Geometry check sheet. Reference: the model listing, model coordinates, mm. Face numbers are marked on the shaded views. A direction names the side the tool comes from. Give positions to 0.01 mm unless a question says otherwise; leave off trailing zeros. Write each loop counter-clockwise with the first axis right and the second up, starting at its lowest first coordinate (ties: lowest second). Pieces come first, ordered by that corner, then holes.
(1) Depth check by flat-ended pin: P1, Ø0.6, axis at y = 10.5, z = 3.5, coming from the -X side; P2, Ø5, axis at x = -6.5, y = 5, coming from the +Z side. Enter the tip coordinate at first touch or a pass-through.
(2) Tool access check on the marked faces 1, 2, 3, 4 and 5. Record the directions out of +Z, -Z, +X, -X, +Y, -Y that give a thin tool (end or side, any length) a straight path to the whole face; none if there is none.
(3) Cross-section at C-C (y = 10.5). Count the separate pieces of the cut face and the enclosed holes in it, and give its area (3 significant figures).
(4) Thickness scan on line 1 along Y through (x, z) = (7.62, 3.35) (3 decimals); line 2 along X through (y, z) = (-4, 2.65); line 3 along X through (y, z) = (8.75, 0.3). Record the ranges inside material, lowest first.
(5) Cross-section at A-A (x = 0). Record the boundary of the cut face in (y, z) (3 decimals), and give its area (3 significant figures).
(6) Cross-section at B-B (y = 0). Record the boundary of the cut face in (x, z).
(7) Mould release check, pull along Y, two halves, no side actions. Record for the marked faces 6, 7 and 8: +Y half, -Y half, draft (parallel to the pull), parting line (faces both ways), or undercut.
(8) Cross-section at D-D (x = -4.25). Record the boundary of the cut face in (y, z) (3 decimals), and give its area (3 significant figures).
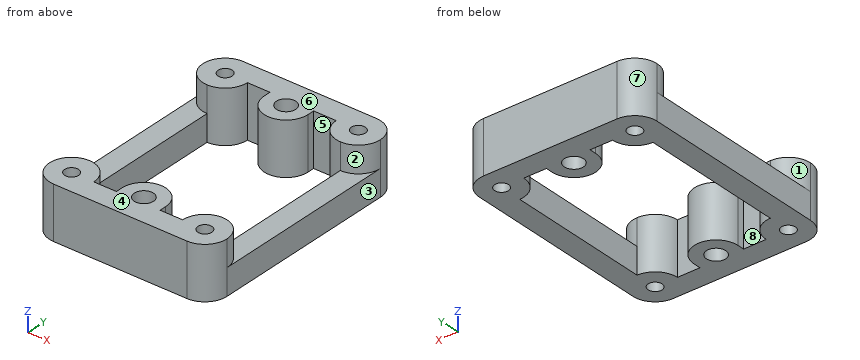
```python
from build123d import *

# Parameters (mm, degrees)
SKETCH_R        = 0.8
PAD_DEPTH       = 6
POCKET_DEPTH    = 6.001
SKETCH002_W     = 22
SKETCH002_H     = 16.5
POCKET001_DEPTH = 3
FILLET_R        = 2.539
PAD001_DEPTH    = 6
SKETCH004_R     = 1.1
POCKET002_DEPTH = 6.001


with BuildPart() as part:
    # Sketch → Pad (new body)
    with BuildSketch(Plane.XY):
        with BuildLine():
            Line((-7.62, 13.335), (7.62, 13.335))
            ThreePointArc((10.16, 10.795), (9.416051, 12.591051), (7.62, 13.335))
            Line((10.16, 10.795), (10.16, -10.795))
            ThreePointArc((7.62, -13.335), (9.416051, -12.591051), (10.16, -10.795))
            Line((7.62, -13.335), (-7.62, -13.335))
            ThreePointArc((-10.16, -10.795), (-9.416051, -12.591051), (-7.62, -13.335))
            Line((-10.16, -10.795), (-10.16, 10.795))
            ThreePointArc((-7.62, 13.335), (-9.416051, 12.591051), (-10.16, 10.795))
        make_face()
        with Locations((-7.62, 10.795)):
            Circle(SKETCH_R, mode=Mode.SUBTRACT)
        with Locations((-7.62, -10.795)):
            Circle(SKETCH_R, mode=Mode.SUBTRACT)
        with Locations((7.62, -10.795)):
            Circle(SKETCH_R, mode=Mode.SUBTRACT)
        with Locations((7.62, 10.795)):
            Circle(SKETCH_R, mode=Mode.SUBTRACT)
    extrude(amount=PAD_DEPTH)

    # Sketch001 (on Face14 of Pad) → Pocket (cut, through all)
    with BuildSketch(Plane.XY.offset(6)):
        with BuildLine():
            Line((-5.08, 10.795), (5.08, 10.795))
            ThreePointArc((5.08, 10.795), (5.823949, 8.998949), (7.62, 8.255))
            Line((7.62, 8.255), (7.62, -8.255))
            ThreePointArc((7.62, -8.255), (5.823949, -8.998949), (5.08, -10.795))
            Line((5.08, -10.795), (-5.08, -10.795))
            ThreePointArc((-5.08, -10.795), (-5.823949, -8.998949), (-7.62, -8.255))
            Line((-7.62, -8.255), (-7.62, 8.255))
            ThreePointArc((-7.62, 8.255), (-5.823949, 8.998949), (-5.08, 10.795))
        make_face()
    extrude(amount=-POCKET_DEPTH, mode=Mode.SUBTRACT)

    # Sketch002 (on Face5 of Pocket) → Pocket001 (cut)
    with BuildSketch(Plane.XY.offset(6)):
        Rectangle(SKETCH002_W, SKETCH002_H)
    extrude(amount=-POCKET001_DEPTH, mode=Mode.SUBTRACT)

    # Fillet
    fillet_edges = [part.edges().sort_by_distance(p)[0] for p in [
        (-10.16, 8.25, 4.5),
        (-10.16, -8.25, 4.5),
        (10.16, 8.25, 4.5),
        (10.16, -8.25, 4.5),
    ]]
    fillet(fillet_edges, radius=FILLET_R)

    # Sketch003 (on Face6 of Fillet) → Pad001 (join)
    with BuildSketch(Plane(origin=(0, 0, 0), x_dir=(1, 0, 0), z_dir=(0, 0, -1))):
        with BuildLine():
            Line((-2.5, 10.8), (2.5, 10.8))
            Line((2.5, 10.8), (2.5, 10))
            ThreePointArc((-2.5, 10), (0, 7.5), (2.5, 10))
            Line((-2.5, 10), (-2.5, 10.8))
        make_face()
        with BuildLine():
            Line((-2.5, -10.8), (2.5, -10.8))
            Line((2.5, -10.8), (2.5, -10))
            ThreePointArc((2.5, -10), (0, -7.5), (-2.5, -10))
            Line((-2.5, -10), (-2.5, -10.8))
        make_face()
    extrude(amount=-PAD001_DEPTH)

    # Sketch004 (on Face44 of Pad001) → Pocket002 (cut, through all)
    with BuildSketch(Plane(origin=(0, 0, 0), x_dir=(1, 0, 0), z_dir=(0, 0, -1))):
        with Locations((0, 10)):
            Circle(SKETCH004_R)
        with Locations((0, -10)):
            Circle(SKETCH004_R)
    extrude(amount=-POCKET002_DEPTH, mode=Mode.SUBTRACT)


solid = part.part
```
Reply:
1. P1: stops at x = -10.16
1. P2: stops at z = 3
2. face 1: +Z, -X
2. face 2: +Z, +X
2. face 3: +Z, -Z, +X, +Y, -Y
2. face 4: +Z, +X, -X, +Y, -Y
2. face 5: +Z, -Z
3. separate pieces: 6
3. enclosed holes: 0
3. area: 61.1 mm2
4. line 1: y = -13.335 to -11.595, -9.995 to -8.255, 8.255 to 9.995, 11.595 to 13.335
4. line 2: x = -10.16 to -7.62, 7.62 to 10.16
4. line 3: x = -10.16 to -6.11, -2.17 to 2.17, 6.11 to 10.16
5. outline: (-13.335, 0) - (-11.1, 0) - (-11.1, 6) - (-13.335, 6) - close; (-8.9, 0) - (-7.5, 0) - (-7.5, 6) - (-8.9, 6) - close; (7.5, 0) - (8.9, 0) - (8.9, 6) - (7.5, 6) - close; (11.1, 0) - (13.335, 0) - (13.335, 6) - (11.1, 6) - close
5. area: 43.6 mm2
6. outline: (-10.16, 0) - (-7.62, 0) - (-7.62, 3) - (-10.16, 3) - close; (7.62, 0) - (10.16, 0) - (10.16, 3) - (7.62, 3) - close
7. face 6: draft
7. face 7: +Y half
7. face 8: undercut
8. outline: (-13.335, 0) - (-10.795, 0) - (-10.795, 6) - (-13.335, 6) - close; (10.795, 0) - (13.335, 0) - (13.335, 6) - (10.795, 6) - close
8. area: 30.5 mm2
